from build123d import *

# Parameters (mm, degrees)
SKETCH1_R           = 4
SKETCH1_R_2         = 3
SKETCH1_R_3         = 3.17
BOSS_EXTRUDE1_DEPTH = 2


with BuildPart() as part:
    # Sketch1 → Boss-Extrude1 (new body)
    with BuildSketch(Plane(origin=(0, 0, 0), x_dir=(0, 0, -1), z_dir=(1, 0, 0))):
        with BuildLine():
            Line((22.098803657, -49.511248032), (22.098803657, -7.511248032))
            Line((22.098803657, -7.511248032), (12.098803657, -7.511248032))
            Line((12.098803657, -7.511248032), (12.098803657, -6.511248032))
            ThreePointArc((12.098803657, -6.511248032), (11.805910438, -5.804141251), (11.098803657, -5.511248032))
            Line((11.098803657, -5.511248032), (-1.901196343, -5.511248032))
            ThreePointArc((-1.901196343, -5.511248032), (-2.608303125, -5.804141251), (-2.901196343, -6.511248032))
            Line((-2.901196343, -6.511248032), (-2.901196343, -7.511248032))
            Line((-2.901196343, -7.511248032), (-7.901196343, -7.511248032))
            Line((-7.901196343, -7.511248032), (-7.901196343, 37.488751968))
            Line((-7.901196343, 37.488751968), (-16.151705215, 37.488751968))
            Line((-16.151705215, 37.488751968), (-16.151705215, 38.488751968))
            ThreePointArc((-16.151705215, 38.488751968), (-16.444598434, 39.195858749), (-17.151705215, 39.488751968))
            Line((-17.151705215, 39.488751968), (-55.650687472, 39.488751968))
            ThreePointArc((-55.650687472, 39.488751968), (-56.357794253, 39.195858749), (-56.650687472, 38.488751968))
            Line((-56.650687472, 38.488751968), (-56.650687472, 37.488751968))
            Line((-56.650687472, 37.488751968), (-60.101196343, 37.488751968))
            Line((-60.101196343, 37.488751968), (-60.101196343, 29.488751968))
            Line((-60.101196343, 29.488751968), (-62.101196343, 29.488751968))
            Line((-62.101196343, 29.488751968), (-62.101196343, 37.488751968))
            Line((-62.101196343, 37.488751968), (-67.901196343, 37.488751968))
            Line((-67.901196343, 37.488751968), (-67.901196343, -49.511248032))
            Line((-67.901196343, -49.511248032), (-56.650687472, -49.511248032))
            Line((-56.650687472, -49.511248032), (-56.650687472, -50.511248032))
            ThreePointArc((-56.650687472, -50.511248032), (-56.357794253, -51.218354813), (-55.650687472, -51.511248032))
            Line((-55.650687472, -51.511248032), (1.848294785, -51.511248032))
            ThreePointArc((1.848294785, -51.511248032), (2.555401566, -51.218354813), (2.848294785, -50.511248032))
            Line((2.848294785, -50.511248032), (2.848294785, -49.511248032))
            Line((2.848294785, -49.511248032), (22.098803657, -49.511248032))
        make_face()
        with Locations((3.81328303, -32.011248032)):
            Circle(SKETCH1_R, mode=Mode.SUBTRACT)
        with Locations((-9.18671697, -19.011248032)):
            Circle(SKETCH1_R_2, mode=Mode.SUBTRACT)
        with Locations((16.81328303, -19.011248032)):
            Circle(SKETCH1_R_2, mode=Mode.SUBTRACT)
        with Locations((16.81328303, -45.011248032)):
            Circle(SKETCH1_R_2, mode=Mode.SUBTRACT)
        with Locations((-9.18671697, -45.011248032)):
            Circle(SKETCH1_R_2, mode=Mode.SUBTRACT)
        with Locations((-52.101196343, -6.011248032)):
            Circle(SKETCH1_R_3, mode=Mode.SUBTRACT)
        with Locations((-24.143956657, -19.011248032)):
            Circle(SKETCH1_R_3, mode=Mode.SUBTRACT)
    extrude(amount=BOSS_EXTRUDE1_DEPTH)


solid = part.part
Geometry check sheet. Reference: the model listing, model coordinates, mm. A direction names the side the tool comes from. Round coordinates to 2 decimals unless told otherwise and drop trailing zeros. Loops run counter-clockwise (first coordinate to the right, second up) from the corner with the lowest first, then second, coordinate; pieces in that order, holes last. Notation, with made-up numbers: (15.25, -1) -> (70.25, -1) arc R24 cw to (70.25, 23) -> close; hole circle Ø7 at (48.25, 87.5). An arc over 180 degrees is marked (long way). Answer as a JSON object with one key per item and string values. Group by question number.
Item 1: Cross-section at B-B, the plane z = 51.5. Record the cut outline in (x, y).
Item 2: Cross-section at C-C, the plane x = 1.2. Count the separate pieces of the cut face and the enclosed holes in it, plus the area to 3 significant figures.
Item 3: Release check for a two-part mould opening along Y. For faces 6 (the face through (0.99, -35.56, -5.66)), 7 (the face through (0.99, -21.94, 9.84)), 8 (the face through (1, -7.511, 5)), 9 (the face through (1, 33, 62.101)) record: pulls with the +Y half, pulls with the -Y half, needs draft (parallel to the pull), parting line crosses it, or undercut.
Item 4: Thickness scan on line 1 along Y through (x, z) = (1.95, 52); line 2 along Z through (x, y) = (1.35, -7); line 3 along Y through (x, z) = (0.5, 10). Record the ranges inside material, lowest first.
Item 5: Depth check by flat-ended pin: pin 1 Ø0.5 at (x, y) = (1, -50) entering from -Z; pin 2 Ø1 at (x, z) = (1.5, 64.5) entering from +Y; pin 3 Ø0.6 at (x, z) = (1, -9) entering from -Y. Enter the tip coordinate at first touch or a pass-through.
Item 6: Cross-section at D-D, the plane y = 11.5. Record the cut outline in (x, z), plus the area to 3 significant figures.
Item 7: Cross-section at A-A, the plane y = -30. Record the cut outline in (x, z), plus the area to 3 significant figures.
Item 8: Set-up check for faces 1 (the face through (1, -29, -22.099)), 2 (the face through (1, 34, 60.101)), 3 (the face through (1, -49.511, -12)), 4 (the face through (1, 37.489, 58)), 5 (the face through (1, 37.489, 12)): record each of +Z, -Z, +X, -X, +Y, -Y from which the full face is reachable in a straight line by a thin tool's end or side.
Determined:
{
 "1": {"outline": "(0, -51.51) -> (2, -51.51) -> (2, -9.12) -> (0, -9.12) -> close; (0, -2.9) -> (2, -2.9) -> (2, 39.49) -> (0, 39.49) -> close"},
 "2": {"separate pieces": "1", "enclosed holes": "7", "area": "6,470 mm²"},
 "3": {"face 6": "undercut", "face 7": "undercut", "face 8": "pulls with the +Y half", "face 9": "needs draft"},
 "4": {"line 1": "y = -51.51 to -9.18, -2.84 to 39.49", "line 2": "z = -12.1 to 2.9, 7.9 to 49.09, 55.11 to 67.9", "line 3": "y = -51.51 to -47.9, -42.12 to -21.9, -16.12 to 37.49"},
 "5": {"pin 1": "stops at z = -2.85", "pin 2": "stops at y = 37.49", "pin 3": "stops at y = -49.51"},
 "6": {"outline": "(0, 7.9) -> (2, 7.9) -> (2, 67.9) -> (0, 67.9) -> close", "area": "120 mm²"},
 "7": {"outline": "(0, -22.1) -> (2, -22.1) -> (2, -7.27) -> (0, -7.27) -> close; (0, -0.36) -> (2, -0.36) -> (2, 67.9) -> (0, 67.9) -> close", "area": "166 mm²"},
 "8": {"face 1": "-Z, +X, -X, +Y, -Y", "face 2": "+X, -X, +Y", "face 3": "-Z, +X, -X, -Y", "face 4": "+Z, +X, -X, +Y", "face 5": "-Z, +X, -X, +Y"}
}
